Here's how the part is built. I have some questions about the finished solid (model axes, mm). A direction names the side the tool comes from. Give positions to 0.01 mm unless a question says otherwise; leave off trailing zeros.
Q1. Will these pins go through, and if not, where does the flat tip stop? P1, Ø2.5, axis at y = 0, z = 31.75, coming from the -X side; P2, Ø1.5, axis at x = 4.5, y = 38, coming from the -Z side; P3, Ø8, axis at x = 12, z = 34.5, coming from the -Y side; P4, Ø1.5, axis at x = 14.5, y = 12, coming from the -Z side.
Q2. For faces 5 (the face through (10.02, 53.97, -0.52)), 6 (the face through (12.7, 0, 7)), which set-ups out of +Z, -Z, +X, -X, +Y, -Y let a thin tool reach every point of the face, with its end or its side?
Q3. We'd pull the mould along Z, two halves only. Please class faces 1 (the face through (16.457, 0.42, -30.418)), 2 (the face through (8.77, -59.51, 13.21)), 3 (the face through (0, -26, -26)), 4 (the face through (10.018, -36.877, -32.552)): +Z half, -Z half, draft (parallel to the pull), parting line (faces both ways), or undercut.
Q4. If we section it at A-A (x = 9): Give the number of separate pieces and of enclosed holes in the cut face, plus the area to 3 significant figures.
Q5. I need wall thicknesses on line 1 (Y direction, x = 16.5, z = 0); line 2 (Y direction, x = 4.5, z = -2.5) (3 decimals); line 3 (Y direction, x = 8.25, z = 2). Which ranges of each line are inside material? Lowest first, please.
from build123d import *

# Parameters (mm, degrees)
SKETCH1_R           = 60.96
BOSS_EXTRUDE1_DEPTH = 20.32
FILLET1_R           = 2.54
SKETCH2_R           = 4.508
CUT_EXTRUDE1_DEPTH  = 6.35
SKETCH4_R           = 6.35
CUT_EXTRUDE3_DEPTH  = 89.572826533
SKETCH5_R           = 3.175
CUT_EXTRUDE4_DEPTH  = 89.572826533
CIRPATTERN2_COUNT   = 8
SKETCH6_R           = 34.925
CUT_EXTRUDE5_DEPTH  = 12.7
SKETCH7_R           = 1.397
CUT_EXTRUDE6_DEPTH  = 7.62


with BuildPart() as part:
    # Sketch1 → Boss-Extrude1 (new body)
    with BuildSketch(Plane(origin=(0, 0, 0), x_dir=(0, 0, -1), z_dir=(1, 0, 0))):
        Circle(SKETCH1_R)
    extrude(amount=BOSS_EXTRUDE1_DEPTH)

    # Fillet1
    fillet1_edges = [part.edges().sort_by_distance(p)[0] for p in [
        (20.32, 0, 60.96),
    ]]
    fillet(fillet1_edges, radius=FILLET1_R)

    # Sketch2 → Cut-Extrude1 (cut)
    with BuildSketch(Plane(origin=(20.32, 0, 0), x_dir=(0, 0, -1), z_dir=(1, 0, 0))):
        Circle(SKETCH2_R)
    extrude(amount=-CUT_EXTRUDE1_DEPTH, mode=Mode.SUBTRACT)

    # Sketch4 → Cut-Extrude3 (cut, through all)
    with BuildSketch(Plane(origin=(20.32, 0, 0), x_dir=(0, 0, -1), z_dir=(1, 0, 0))):
        Circle(SKETCH4_R)
    extrude(amount=-CUT_EXTRUDE3_DEPTH, mode=Mode.SUBTRACT)

    # Sketch5 → Cut-Extrude4 (cut, through all)
    with BuildSketch(Plane.ZY):
        with Locations((-36.188764222, 35.651274088)):
            Circle(SKETCH5_R)
    cut_extrude4 = extrude(amount=-CUT_EXTRUDE4_DEPTH, mode=Mode.SUBTRACT)

    # CirPattern2: Cut-Extrude4 ×8 about axis, 1 skipped
    cirpattern2_axis = Axis((0, 0, 0), (1, 0, 0))
    add([cut_extrude4.rotate(cirpattern2_axis, i * 360 / CIRPATTERN2_COUNT) for i in range(1, CIRPATTERN2_COUNT) if i not in (7,)], mode=Mode.SUBTRACT)

    # Sketch6 → Cut-Extrude5 (cut)
    with BuildSketch(Plane.ZY):
        Circle(SKETCH6_R)
    extrude(amount=-CUT_EXTRUDE5_DEPTH, mode=Mode.SUBTRACT)

    # Sketch7 → Cut-Extrude6 (cut)
    with BuildSketch(Plane.ZY.offset(-12.7)):
        with Locations((0, 31.75)):
            Circle(SKETCH7_R)
        with Locations((31.75, 0)):
            Circle(SKETCH7_R)
        with Locations((0, -31.75)):
            Circle(SKETCH7_R)
        with Locations((-31.75, 0)):
            Circle(SKETCH7_R)
    extrude(amount=-CUT_EXTRUDE6_DEPTH, mode=Mode.SUBTRACT)


solid = part.part
Check sheet entries:
1. P1: passes through
1. P2: stops at z = -48.26
1. P3: stops at y = -52.78
1. P4: stops at z = -59.91
2. face 5: +X, -X
2. face 6: -X
3. face 1: undercut
3. face 2: parting line
3. face 3: draft
3. face 4: undercut
4. separate pieces: 1
4. enclosed holes: 8
4. area: 7,620 mm2
5. line 1: y = -60.96 to -53.95, -47.65 to -33.15, -30.35 to -6.35, 6.35 to 30.35, 33.15 to 47.65, 53.95 to 60.96
5. line 2: y = -60.909 to -52.135, -49.462 to -34.835, 34.835 to 48.435, 53.162 to 60.909
5. line 3: y = -60.93 to -53.53, -48.07 to -34.87, 34.87 to 48.7, 52.9 to 60.93
